Source: CAD feature listing. Evaluate the final solid. Frame: model axes, mm. Face numbers are marked on the shaded views. A direction names the side the tool comes from. Coordinates: 2 decimals unless noted, no trailing zeros. Loops run counter-clockwise (first coordinate to the right, second up) from the corner with the lowest first, then second, coordinate; pieces in that order, holes last.
Item 1: Section query A-A, the plane y = -17.5. Return the cut outline in (x, z) (3 decimals), then the cut area to 3 significant figures.
Item 2: Line query: probe 1 along Z at (x, y) = (0, 9); probe 2 along Z at (x, y) = (4, -6); probe 3 along Z at (x, y) = (-8.5, -5.5). Output: solid intervals per line, ascending.
Item 3: Pin query (flat end, axial travel): pin 1 Ø2.5 at (y, z) = (8.5, 0) entering from +X; pin 2 Ø6 at (y, z) = (12.5, -4.5) entering from +X; pin 3 Ø6 at (x, y) = (-10.5, 0) entering from -Z. Return the tip coordinate at first contact, or that it passes through.
Item 4: Section query C-C, the plane y = 4.5. Return the cut outline in (x, z), then the cut area to 3 significant figures.
Item 5: Reachability of the marked faces 1 and 2 from +Z, -Z, +X, -X, +Y, -Y: full face, straight path, thin tool, end or side. Return the list, or none.
Item 6: Section query B-B, the plane z = 0. State how many separate pieces and enclosed holes the cut face has, then the cut area to 3 significant figures.
Item 7: Pull-direction query (X, two-part tool) for the marked faces 3, 4 and 5; classes: +X half, -X half, draft (parallel to the pull), parting line (faces both ways), or undercut.
Autodesk Inventor part; units mm, degrees
ref_plane "XZ Plane" through (0, 0, 0) normal (0, 1, 0) x (-1, 0, 0)
ref_plane "XY Plane" through (0, 0, 0) normal (0, 0, 1) x (1, 0, 0)
sketch "Sketch1" plane through (0, 0, 0) normal (0, 1, 0) x (-1, 0, 0)
  circle A0 centre (0, 0) radius 3.2318
  line L0 (2.28, 2.2905) -> (2.28, -2.2905)
  circle A1 centre (0, 0) radius 10.5918
  dimension "d2" = 5.5118
  dimension "d3" = 21.1836
extrude "Extrusion1" add sketch "Sketch1" along normal blind 18.034 contours A0 L0 | A1 picked at (2.4147, -0.6)
sketch "Sketch2" plane through (0, 0, 0) normal (0, -1, 0) x (1, 0, 0)
  circle A0 centre (0, 0) radius 15.24
  dimension "d6" = 30.48
extrude "Extrusion2" add sketch "Sketch2" along normal blind 2.54
sketch "Sketch3" plane through (0, -2.54, 0) normal (0, -1, 0) x (1, 0, 0)
  circle A0 centre (0, 0) radius 14.351
  circle A1 centre (0, 0) radius 16.4291
  dimension "d9" = 28.702
extrude "Extrusion3" add sketch "Sketch3" along normal blind 20.32
fillet "Fillet3" radius 2.54 1 edges at (10.5918, 0, 0)
fillet "Fillet4" radius 2.54 1 edges at (-15.24, -2.54, 0)
fillet "Fillet5" radius 2.54 1 edges at (-15.24, 0, 0)
ref_plane "Work Plane1" through (12.7, 0, 0) normal (1, 0, 0) x (0, 1, 0)
sketch "Sketch6" plane through (12.7, 0, 0) normal (1, 0, 0) x (0, 1, 0)
  arc A0 (-8.3185, -1.27) -> (-8.3185, 1.27) centre (-8.3185, 0) ccw construction
  arc A1 (-18.4785, 1.27) -> (-18.4785, -1.27) centre (-18.4785, 0) ccw construction
  line L0 (-18.4785, 1.27) -> (-8.3185, 1.27) construction
  line L1 (-8.3185, -1.27) -> (-18.4785, -1.27) construction
  arc A2 (-8.3185, -3.175) -> (-8.3185, 3.175) centre (-8.3185, 0) ccw
  line L2 (-8.3185, -3.175) -> (-18.4785, -3.175)
  arc A3 (-18.4785, 3.175) -> (-18.4785, -3.175) centre (-18.4785, 0) ccw
  line L3 (-18.4785, 3.175) -> (-8.3185, 3.175)
  point P0 (0, 0)
  dimension "d34" = 3.175
extrude "Extrusion6" cut sketch "Sketch6" along normal blind 25.4
mirror "Mirror1" about plane through (0, 0, 0) normal (1, 0, 0) of "Extrusion6"
fillet "Fillet10" radius 0.762 1 edges at (-16.4291, -22.86, 0)
sketch "Sketch7" plane through (0, -2.54, 0) normal (0, -1, 0) x (1, 0, 0)
  circle A0 centre (0, 0) radius 12.7
  dimension "d40" = 25.4
extrude "Extrusion7" add sketch "Sketch7" along normal blind 20.32
sketch "Sketch8" plane through (0, -22.86, 0) normal (0, -1, 0) x (1, 0, 0)
  line L0 (-0.4572, 8.89) -> (0.4572, 8.89)
  line L1 (0.4572, 8.89) -> (0.4572, -8.89)
  line L2 (0.4572, -8.89) -> (-0.4572, -8.89)
  line L3 (-0.4572, -8.89) -> (-0.4572, 8.89)
  line L4 (-0.4572, 8.89) -> (0.4572, -8.89) construction
  line L5 (0.4572, 8.89) -> (-0.4572, -8.89) construction
  point P0 (0, 0)
  dimension "d43" = 0.9144
  dimension "d44" = 17.78
extrude "Extrusion8" cut sketch "Sketch8" against normal blind 20.32
properties part number "Autofeeder part 1"
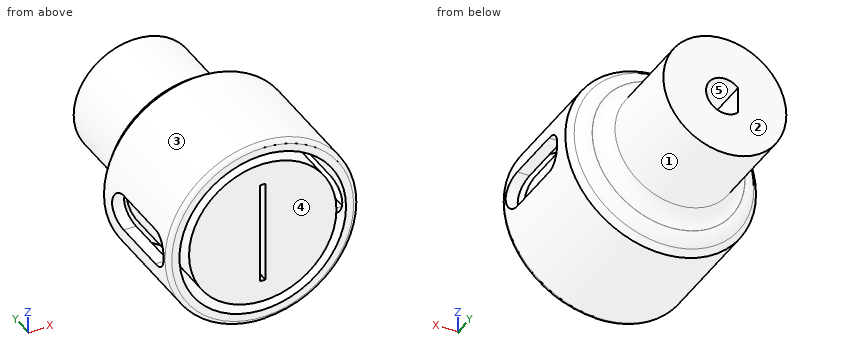
Verdict:
1. outline: (-16.119, -3.175) arc R16.429 ccw to (16.119, -3.175) - (13.995, -3.175) arc R14.351 cw to (-13.995, -3.175) - close; (-16.119, 3.175) - (-13.995, 3.175) arc R14.351 cw to (13.995, 3.175) - (16.119, 3.175) arc R16.429 ccw to start; circle Ø25.4 at (0, 0); hole (-0.457, -8.89) - (0.457, -8.89) - (0.457, 8.89) - (-0.457, 8.89) - close
1. area: 665 mm2
2. probe 1: z = -10.59 to -3.23, 3.23 to 10.59
2. probe 2: z = -15.93 to -13.78, -12.05 to 12.05, 13.78 to 15.93
2. probe 3: z = -14.06 to -11.56, -9.44 to 9.44, 11.56 to 14.06
3. pin 1: stops at x = 10.59
3. pin 2: stops at x = 10.49
3. pin 3: stops at z = -13.81
4. outline: circle Ø21.18 at (0, 0); hole (-2.28, -2.29) arc R3.23 ccw (long way) to (-2.28, 2.29) - close
4. area: 323 mm2
5. face 1: +Y
5. face 2: +Z, -Z, +X, -X, +Y
6. separate pieces: 3
6. enclosed holes: 0
6. area: 876 mm2
7. face 3: parting line
7. face 4: draft
7. face 5: undercut
